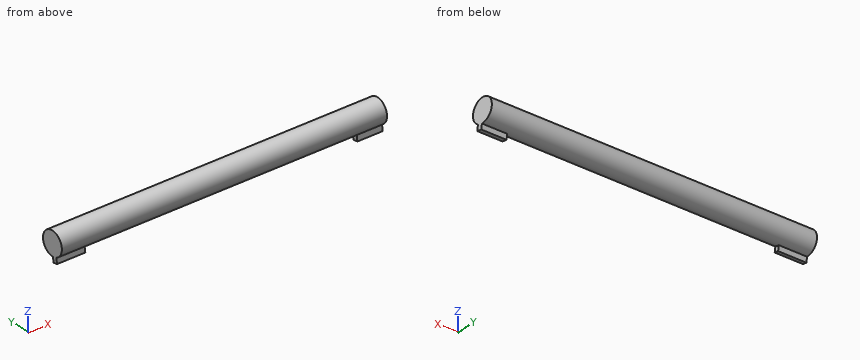
from build123d import *

# Parameters (mm, degrees)
SKETCH1_R             = 7
BOSS_EXTRUDE1_DEPTH   = 192.48
SKETCH2_W             = 15
SKETCH2_H             = 3
BOSS_EXTRUDE2_DEPTH   = 3
SKETCH2_W_2           = 16.730233444
SKETCH2_H_2           = 2.564845708
BOSS_EXTRUDE2_2_DEPTH = 3
SKETCH3_W             = 16.730233444
SKETCH3_H             = 2.564845708
BOSS_EXTRUDE3_DEPTH   = 10
SKETCH4_W             = 15
SKETCH4_H             = 3
BOSS_EXTRUDE4_DEPTH   = 10


with BuildPart() as part:
    # Sketch1 → Boss-Extrude1 (new body)
    with BuildSketch(Plane(origin=(0, 0, 0), x_dir=(0, 0, -1), z_dir=(1, 0, 0))):
        Circle(SKETCH1_R)
    extrude(amount=BOSS_EXTRUDE1_DEPTH)



with BuildPart() as body_2:
    # Sketch2 → Boss-Extrude2 (new body)
    with BuildSketch(Plane(origin=(0, -1.130854734, -6.908050924), x_dir=(1, 0, 0), z_dir=(0, -0.161550676, -0.986864418))):
        with Locations((184.98, 0.763298878)):
            Rectangle(SKETCH2_W, SKETCH2_H)
    extrude(amount=BOSS_EXTRUDE2_DEPTH)


with BuildPart() as body_3:
    # Sketch2 → Boss-Extrude2 2 (new body)
    with BuildSketch(Plane(origin=(0, -1.130854734, -6.908050924), x_dir=(1, 0, 0), z_dir=(0, -0.161550676, -0.986864418))):
        with Locations((8.365116722, 0.545721732)):
            Rectangle(SKETCH2_W_2, SKETCH2_H_2)
    extrude(amount=BOSS_EXTRUDE2_2_DEPTH)


with BuildPart() as part_1:
    add(part.part)

    add(body_3.part)  # Boss-Extrude3 merges body 3
    # Sketch3 → Boss-Extrude3 (add)
    with BuildSketch(Plane(origin=(0, -1.130854734, -6.908050924), x_dir=(1, 0, 0), z_dir=(0, 0.161550676, 0.986864418))):
        with Locations((8.365116722, -0.545721732)):
            Rectangle(SKETCH3_W, SKETCH3_H)
    extrude(amount=BOSS_EXTRUDE3_DEPTH)


    add(body_2.part)  # Boss-Extrude4 merges body 2
    # Sketch4 → Boss-Extrude4 (add)
    with BuildSketch(Plane(origin=(0, -1.130854734, -6.908050924), x_dir=(1, 0, 0), z_dir=(0, 0.161550676, 0.986864418))):
        with Locations((184.98, -0.763298878)):
            Rectangle(SKETCH4_W, SKETCH4_H)
    extrude(amount=BOSS_EXTRUDE4_DEPTH)


solid = part_1.part
Design review of the part built by this model. Coordinates are the model's own, in mm. Coordinates: 2 decimals unless noted, no trailing zeros. Order: outer loops, then holes, each group sorted by start corner. A loop starts at its lowest first (then second) coordinate and runs counter-clockwise, first axis right, second up. Notation, with made-up numbers: (-13.75, 26.25) -> (18.25, 26.25) arc R27 ccw to (18.25, 48.25) -> close; hole circle Ø8 at (-34.75, 50.25). An arc over 180 degrees is marked (long way). One line per item, written item: value.
1) We need section C-C, the plane y = 2.75. Give the boundary of the cut face in (x, z).
Output values:
outline: (0, -6.44) -> (192.48, -6.44) -> (192.48, 6.44) -> (0, 6.44) -> close
2) To check wall thickness, follow probe 1 along X at (y, z) = (-1.25, -9.5); probe 2 along Y at (x, z) = (26, -0.5). State the ranges of each line that lie inside material, in increasing order. Write a range as [from, to].
Output values:
probe 1: x = [0, 16.73], [177.48, 192.48]
probe 2: y = [-6.98, 6.98]
3) We need section A-A, the plane x = 154. Give the boundary of the cut face in (y, z), then the cut area to 3 significant figures.
Output values:
outline: circle Ø14 at (0, 0)
area: 154 mm2
4) Clearance check with flat-ended pins moving along their axes: P1, Ø2, axis at x = 22.5, y = 3.5, coming from the -Z side; P2, Ø4, axis at y = -1.5, z = -7.5, coming from the -X side; P3, Ø6, axis at x = 85, y = 5.5, coming from the +Z side; P4, Ø8, axis at x = 103.5, y = -0.5, coming from the -Z side. State where each tip first meets the part, or that it passes through.
Output values:
P1: stops at z = -6.54
P2: stops at x = 0
P3: stops at z = 6.54
P4: stops at z = -7
5) We need section B-B, the plane z = 1.5. Give the boundary of the cut face in (x, y).
Output values:
outline: (0, -6.84) -> (192.48, -6.84) -> (192.48, 6.84) -> (0, 6.84) -> close
